Here's how the part is built. I have some questions about the finished solid (model axes, mm). A direction names the side the tool comes from. Round coordinates to 2 decimals unless told otherwise and drop trailing zeros. Order: outer loops, then holes, each group sorted by start corner. A loop starts at its lowest first (then second) coordinate and runs counter-clockwise, first axis right, second up. Notation, with made-up numbers: (81.5, 86) -> (133.5, 86) arc R24 ccw to (133.5, 106) -> close; hole circle Ø1 at (8, 84.25). An arc over 180 degrees is marked (long way). Use a Markdown table: item, result. Add a question column.
from build123d import *

# Parameters (mm, degrees)
SKETCH1_R           = 1.5
SKETCH1_R_2         = 1.4224
BOSS_EXTRUDE1_DEPTH = 4
SKETCH2_R           = 3.5
SKETCH2_R_2         = 1.4224
BOSS_EXTRUDE2_DEPTH = 6


with BuildPart() as part:
    # Sketch1 → Boss-Extrude1 (new body)
    with BuildSketch(Plane.XY.offset(189.266714263)):
        with BuildLine():
            Line((108.526557277, 109.730165261), (160.526557277, 109.730165261))
            ThreePointArc((160.526557277, 109.730165261), (163.001431011, 110.755291526), (164.026557277, 113.230165261))
            Line((164.026557277, 113.230165261), (164.026557277, 189.230165261))
            ThreePointArc((164.026557277, 189.230165261), (163.001431011, 191.705038995), (160.526557277, 192.730165261))
            Line((160.526557277, 192.730165261), (108.526557277, 192.730165261))
            ThreePointArc((108.526557277, 192.730165261), (106.051683543, 191.705038995), (105.026557277, 189.230165261))
            Line((105.026557277, 189.230165261), (105.026557277, 113.230165261))
            ThreePointArc((105.026557277, 113.230165261), (106.051683543, 110.755291526), (108.526557277, 109.730165261))
        make_face()
        with Locations((134.526557277, 124.637085275)):
            Circle(SKETCH1_R, mode=Mode.SUBTRACT)
        with Locations((109.526557277, 134.637085275)):
            Circle(SKETCH1_R, mode=Mode.SUBTRACT)
        with Locations((124.526557277, 134.637085275)):
            Circle(SKETCH1_R, mode=Mode.SUBTRACT)
        with Locations((159.526557277, 134.637085275)):
            Circle(SKETCH1_R, mode=Mode.SUBTRACT)
        with Locations((144.526557277, 134.637085275)):
            Circle(SKETCH1_R, mode=Mode.SUBTRACT)
        with Locations((134.526557277, 139.637085275)):
            Circle(SKETCH1_R, mode=Mode.SUBTRACT)
        with Locations((134.526557277, 154.637085275)):
            Circle(SKETCH1_R, mode=Mode.SUBTRACT)
        with Locations((134.526557277, 169.637085275)):
            Circle(SKETCH1_R, mode=Mode.SUBTRACT)
        with Locations((134.526557277, 184.637085275)):
            Circle(SKETCH1_R, mode=Mode.SUBTRACT)
        with Locations((108.526557277, 189.230165261)):
            Circle(SKETCH1_R_2, mode=Mode.SUBTRACT)
        with Locations((160.526557277, 189.230165261)):
            Circle(SKETCH1_R_2, mode=Mode.SUBTRACT)
        with Locations((160.526557277, 113.230165261)):
            Circle(SKETCH1_R_2, mode=Mode.SUBTRACT)
        with Locations((108.526557277, 113.230165261)):
            Circle(SKETCH1_R_2, mode=Mode.SUBTRACT)
    extrude(amount=BOSS_EXTRUDE1_DEPTH)

    # Sketch2 → Boss-Extrude2 (add)
    with BuildSketch(Plane.XY.offset(193.266714263)):
        with Locations((108.526557277, 189.230165261)):
            Circle(SKETCH2_R)
        with Locations((108.526557277, 189.230165261)):
            Circle(SKETCH2_R_2, mode=Mode.SUBTRACT)
        with Locations((160.526557277, 189.230165261)):
            Circle(SKETCH2_R)
        with Locations((160.526557277, 189.230165261)):
            Circle(SKETCH2_R_2, mode=Mode.SUBTRACT)
        with Locations((108.526557277, 113.230165261)):
            Circle(SKETCH2_R)
        with Locations((108.526557277, 113.230165261)):
            Circle(SKETCH2_R_2, mode=Mode.SUBTRACT)
        with Locations((160.526557277, 113.230165261)):
            Circle(SKETCH2_R)
        with Locations((160.526557277, 113.230165261)):
            Circle(SKETCH2_R_2, mode=Mode.SUBTRACT)
    extrude(amount=BOSS_EXTRUDE2_DEPTH)


solid = part.part
(1) I want a section at B-B on x = 114. List the corners of the cut face in (y, z) for me, and give its area (3 significant figures).
(2) If we mould it in two halves opening along X, with no side actions, what happens to faces 3 (the flat face through (105.027, 152, 191)), 4 (the flat face through (134, 109.73, 191)), 5 (the cylindrical face through (159.201, 133.173, 191.239))? For each: pulls with the +X half, pulls with the -X half, needs draft (parallel to the pull), parting line crosses it, or undercut.
(3) On a 3-axis mill with a long thin cutter (end or side, diameter ignored), from which of +Z, -Z, +X, -X, +Y, -Y can I reach the whole of each face in a straight line? I mean faces 1 (the flat face through (134, 152, 193.267)), 2 (the cylindrical face through (145.91, 134.06, 191.24)). Say none if no direction works.
(4) I want a section at C-C on y = 122. List the corners of the cut face in (x, z) for me, and give its area (3 significant figures).
(5) I want a section at A-A on z = 194.5. List the corners of the cut face in (x, y) for me.
(6) Please list where these lines run through material, in increasing order: probe 1 along Z at (x, y) = (148, 154); probe 2 along X at (y, z) = (186, 194); probe 3 along X at (y, z) = (115.5, 193.5). Write a range as from..to.
(7) I'm going to push a flat-ended pin straight in: P1, Ø5, axis at x = 134.53, y = 139.64, coming from the +Z side. Where does the tip first touch, or does it pass through?
Output:
| question | item | result |
|---|---|---|
| 1 | outline | (109.73, 189.27) -> (192.73, 189.27) -> (192.73, 193.27) -> (109.73, 193.27) -> close |
| 1 | area | 332 mm² |
| 2 | face 3 | pulls with the -X half |
| 2 | face 4 | needs draft |
| 2 | face 5 | undercut |
| 3 | face 1 | +Z |
| 3 | face 2 | +Z, -Z |
| 4 | outline | (105.03, 189.27) -> (164.03, 189.27) -> (164.03, 193.27) -> (105.03, 193.27) -> close |
| 4 | area | 236 mm² |
| 5 | outline | circle Ø7 at (108.53, 113.23); circle Ø7 at (108.53, 189.23); circle Ø7 at (160.53, 113.23); circle Ø7 at (160.53, 189.23); hole circle Ø2.84 at (108.53, 113.23); hole circle Ø2.84 at (108.53, 189.23); hole circle Ø2.84 at (160.53, 113.23); hole circle Ø2.84 at (160.53, 189.23) |
| 6 | probe 1 | 189.27..193.27 |
| 6 | probe 2 | 107.18..109.87, 159.18..161.87 |
| 6 | probe 3 | 105.86..111.19, 157.86..163.19 |
| 7 | P1 | z = 193.27 |
